For this review, take the finished solid that the model builds, in its own axes (mm). Coordinates: 2 decimals unless noted, no trailing zeros. Write each loop counter-clockwise with the first axis right and the second up, starting at its lowest first coordinate (ties: lowest second). Pieces come first, ordered by that corner, then holes.
1) We need section B-B on x = -25.4. Write out the cut boundary in (y, z) (3 decimals).
2) We need section A-A on z = -17.78. Write out the cut boundary in (x, y) (3 decimals), then the cut area to 3 significant figures.
3) We need section D-D on x = 68.58. Write out the cut boundary in (y, z) (3 decimals), then the cut area to 3 significant figures.
4) To check wall thickness, follow line 1 along X through (y, z) = (0.55, -34.29) (3 decimals); line 2 along X through (y, z) = (1.65, 2.54) (3 decimals); line 3 along Z through (x, y) = (41.5, 0.1). State the ranges of each line that lie inside material, in increasing order.
5) We need section C-C on z = 2.54. Write out the cut boundary in (x, y) (3 decimals), then the cut area to 3 significant figures.
6) Insertion check: P1, Ø0.7, axis at y = 1, z = 14, coming from the -X side; P2, Ø1.2, axis at x = 55, y = 0.5, coming from the +Z side. Each pin has a flat end and moves straight along its axis. Give the tip position at first contact, or say it passes through.
from build123d import *

# Parameters (mm, degrees)
BOSS_EXTRUDE1_DEPTH = 2.38125
SKETCH3_W           = 38.1
SKETCH3_H           = 50.8
SKETCH3_R           = 1.905
BOSS_EXTRUDE4_DEPTH = 2.38125
SKETCH7_W           = 33.02
SKETCH7_H           = 50.8
CUT_EXTRUDE3_DEPTH  = 3.38125
SKETCH8_R           = 1.905
CUT_EXTRUDE4_DEPTH  = 3.38125


with BuildPart() as part:
    # Sketch1 → Boss-Extrude1 (new body)
    with BuildSketch(Plane(origin=(0, 0, 0), x_dir=(1, 0, 0), z_dir=(0, 1, 0))):
        Polygon((107.95, -12.7), (107.95, 0), (107.95, 38.1), (60.905597294, 38.1), (60.905597294, 31.496), (62.977716984, 31.496), (62.977716984, 28.956), (60.945716984, 28.956), (60.945716984, 21.336), (58.151716984, 21.336), (58.151716984, 28.956), (56.119716984, 28.956), (56.119716984, 31.496), (58.07075, 31.496), (58.07075, 38.1), (52.8955, 38.1), (52.8955, 41.402), (45.72, 41.402), (45.72, 38.1), (40.54475, 38.1), (40.54475, 31.496), (42.57675, 31.496), (42.57675, 28.956), (40.82869895, 28.956), (40.82869895, 21.336), (37.75075, 21.336), (37.75075, 28.956), (35.71875, 28.956), (35.71875, 31.496), (37.75075, 31.496), (37.75075, 38.1), (32.5755, 38.1), (32.5755, 41.402), (25.4, 41.402), (25.4, 38.1), (6.35, 38.1), (6.35, -12.7), (25.4, -12.7), (25.4, -16.002), (32.5755, -16.002), (32.5755, -12.7), (37.75075, -12.7), (37.75075, -6.096), (35.71875, -6.096), (35.71875, -3.556), (37.75075, -3.556), (37.75075, 4.064), (40.82869895, 4.064), (40.82869895, -3.556), (42.57675, -3.556), (42.57675, -6.096), (40.54475, -6.096), (40.54475, -12.7), (45.72, -12.7), (45.72, -16.002), (52.8955, -16.002), (52.8955, -12.7), (58.07075, -12.7), (58.07075, -6.096), (56.119716984, -6.096), (56.119716984, -3.556), (58.151716984, -3.556), (58.151716984, 4.064), (60.945716984, 4.064), (60.945716984, -3.556), (62.977716984, -3.556), (62.977716984, -6.096), (60.86475, -6.096), (60.86475, -12.7), (66.04, -12.7), (73.2155, -12.7), (78.035770588, -12.7), (80.829770588, -12.7), align=None)
    extrude(amount=BOSS_EXTRUDE1_DEPTH)

    # Sketch3 → Boss-Extrude4 (add)
    with BuildSketch(Plane(origin=(0, 2.38125, 0), x_dir=(1, 0, 0), z_dir=(0, 1, 0))):
        with Locations((-12.7, 12.7)):
            Rectangle(SKETCH3_W, SKETCH3_H)
        with Locations((-25.4, -8.89)):
            Circle(SKETCH3_R, mode=Mode.SUBTRACT)
        with Locations((-25.4, 5.08)):
            Circle(SKETCH3_R, mode=Mode.SUBTRACT)
        with Locations((-25.4, 17.78)):
            Circle(SKETCH3_R, mode=Mode.SUBTRACT)
        with Locations((-25.4, 34.29)):
            Circle(SKETCH3_R, mode=Mode.SUBTRACT)
    extrude(amount=-BOSS_EXTRUDE4_DEPTH)

    # Sketch7 → Cut-Extrude3 (cut, through all)
    with BuildSketch(Plane(origin=(0, 2.38125, 0), x_dir=(1, 0, 0), z_dir=(0, 1, 0))):
        with Locations((91.44, 12.7)):
            Rectangle(SKETCH7_W, SKETCH7_H)
    extrude(amount=-CUT_EXTRUDE3_DEPTH, mode=Mode.SUBTRACT)

    # Sketch8 → Cut-Extrude4 (cut, through all)
    with BuildSketch(Plane(origin=(0, 2.38125, 0), x_dir=(1, 0, 0), z_dir=(0, 1, 0))):
        with Locations((68.58, -2.54)):
            Circle(SKETCH8_R)
        with Locations((68.58, 27.94)):
            Circle(SKETCH8_R)
    extrude(amount=-CUT_EXTRUDE4_DEPTH, mode=Mode.SUBTRACT)


solid = part.part
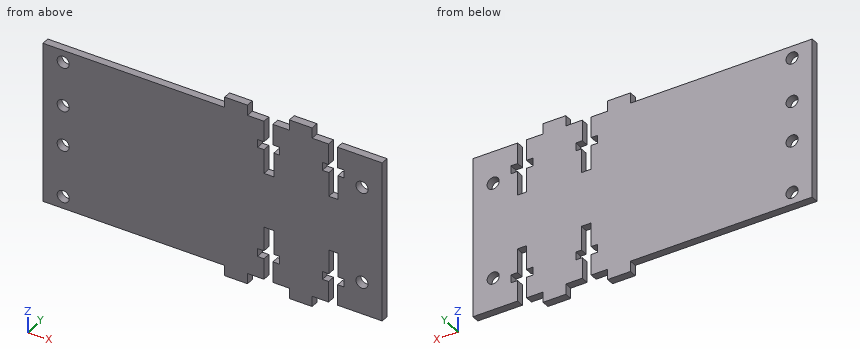
Result:
1. outline: (0, -38.1) - (2.381, -38.1) - (2.381, -36.195) - (0, -36.195) - close; (0, -32.385) - (2.381, -32.385) - (2.381, -19.685) - (0, -19.685) - close; (0, -15.875) - (2.381, -15.875) - (2.381, -6.985) - (0, -6.985) - close; (0, -3.175) - (2.381, -3.175) - (2.381, 6.985) - (0, 6.985) - close; (0, 10.795) - (2.381, 10.795) - (2.381, 12.7) - (0, 12.7) - close
2. outline: (-31.75, 0) - (-27.305, 0) - (-27.305, 2.381) - (-31.75, 2.381) - close; (-23.495, 0) - (74.93, 0) - (74.93, 2.381) - (-23.495, 2.381) - close
2. area: 245 mm2
3. outline: (0, -38.1) - (2.381, -38.1) - (2.381, -29.845) - (0, -29.845) - close; (0, -26.035) - (2.381, -26.035) - (2.381, 0.635) - (0, 0.635) - close; (0, 4.445) - (2.381, 4.445) - (2.381, 12.7) - (0, 12.7) - close
3. area: 103 mm2
4. line 1: x = -31.75 to -27.305, -23.495 to 37.751, 40.545 to 58.071, 60.906 to 74.93
4. line 2: x = -31.75 to 37.751, 40.829 to 58.152, 60.946 to 66.675, 70.485 to 74.93
4. line 3: z = -38.1 to -31.5, -28.96 to 3.56, 6.1 to 12.7
5. outline: (-31.75, 0) - (37.751, 0) - (37.751, 2.381) - (-31.75, 2.381) - close; (40.829, 0) - (58.152, 0) - (58.152, 2.381) - (40.829, 2.381) - close; (60.946, 0) - (66.675, 0) - (66.675, 2.381) - (60.946, 2.381) - close; (70.485, 0) - (74.93, 0) - (74.93, 2.381) - (70.485, 2.381) - close
5. area: 231 mm2
6. P1: stops at x = 25.4
6. P2: stops at z = 12.7
